```python
from build123d import *

# Parameters (mm, degrees)
SZKIC1_R                    = 4.5
DODANIE_WYCI_GNI_CIE1_DEPTH = 10
SZKIC3_R                    = 6.5
WYTNIJ_WYCI_GNI_CIE9_DEPTH  = 6.85
DODANIE_WYCI_GNI_CIE2_DEPTH = 18
DODANIE_WYCI_GNI_CIE3_DEPTH = 31.65
DODANIE_WYCI_GNI_CIE4_DEPTH = 20.5
WYTNIJ_WYCI_GNI_CIE3_REACH  = 73.312
SZKIC8_R                    = 1.7500000000000036
SZKIC8_R_2                  = 1.7499999999999982
SFAZOWANIE1_SIZE            = 2
DODANIE_WYCI_GNI_CIE5_DEPTH = 10
WYTNIJ_WYCI_GNI_CIE4_REACH  = 76.066
SZKIC12_R                   = 1.6000000000000019
WYTNIJ_WYCI_GNI_CIE6_START  = -5
SZKIC14_R                   = 7.499999999999999
WYTNIJ_WYCI_GNI_CIE6_DEPTH  = 5
SZKIC13_R                   = 4.000000000000001
WYTNIJ_WYCI_GNI_CIE5_DEPTH  = 1
ZAOKR_GLENIE1_R             = 2
ZAOKR_GLENIE2_R             = 1
WYTNIJ_WYCI_GNI_CIE7_DEPTH  = 13
WYTNIJ_WYCI_GNI_CIE8_REACH  = 71.325
SZKIC16_R                   = 1.599999999999998


with BuildPart() as part:
    # Szkic1 → Dodanie-wyciągnięcie1 (new body)
    with BuildSketch(Plane(origin=(0, 0, 0), x_dir=(1, 0, 0), z_dir=(0, 1, 0))):
        Polygon((-39.699999999999996, 14.25), (11.950000000000069, 14.25), (18.7, 7.5), (18.7, -7.5), (11.95000000000007, -14.25), (-39.699999999999996, -14.25), align=None)
        with Locations(Location((0, 0, 0), (0, 0, 270))):
            Circle(SZKIC1_R, mode=Mode.SUBTRACT)
    extrude(amount=DODANIE_WYCI_GNI_CIE1_DEPTH)

    # Szkic3 → Wytnij-wyciągnięcie9 (cut)
    with BuildSketch(Plane.XZ):
        with Locations(Location((0, 0, 0), (0, 0, 270))):
            Circle(SZKIC3_R)
    extrude(amount=-WYTNIJ_WYCI_GNI_CIE9_DEPTH, mode=Mode.SUBTRACT)

    # Szkic4 → Dodanie-wyciągnięcie2 (add)
    with BuildSketch(Plane(origin=(0, 10, 0), x_dir=(1, 0, 0), z_dir=(0, 1, 0))):
        Polygon((-39.699999999999996, 14.25), (-15, 14.25), (-14.999999999999996, -14.25), (-39.699999999999996, -14.25), align=None)
    extrude(amount=DODANIE_WYCI_GNI_CIE2_DEPTH)

    # Szkic6 → Dodanie-wyciągnięcie3 (add)
    with BuildSketch(Plane(origin=(0, 27.999999999999996, 0), x_dir=(1, 0, 0), z_dir=(0, 1, 0))):
        Polygon((-39.699999999999996, 14.25), (18.699999999999996, 14.25), (18.7, 10.25), (-39.699999999999996, 10.25), align=None)
    extrude(amount=DODANIE_WYCI_GNI_CIE3_DEPTH)

    # Szkic7 → Dodanie-wyciągnięcie4 (add)
    with BuildSketch(Plane.XY.offset(-10.25)):
        Polygon((18.7, 57.49999999999999), (10.499999999999995, 57.49999999999999), (10.499999999999996, 47.49999999999999), (18.7, 47.49999999999999), align=None)
        Polygon((-39.699999999999996, 57.499999999999986), (-31.000000000000007, 57.499999999999986), (-31.000000000000004, 47.499999999999986), (-39.699999999999996, 47.499999999999986), align=None)
    extrude(amount=DODANIE_WYCI_GNI_CIE4_DEPTH)

    # Szkic8 → Wytnij-wyciągnięcie3 (cut, up to next)
    with BuildSketch(Plane(origin=(0, 57.499999999999986, 0), x_dir=(1, 0, 0), z_dir=(0, 1, 0)), mode=Mode.PRIVATE) as wytnij_wyci_gni_cie3_sk1:
        with Locations(Location((-34.5, 5.450000000000001, 0), (0, 0, 270))):
            Circle(SZKIC8_R)
    wytnij_wyci_gni_cie3_tool1 = extrude(wytnij_wyci_gni_cie3_sk1.sketch, amount=-WYTNIJ_WYCI_GNI_CIE3_REACH, mode=Mode.PRIVATE) & part.part
    # Szkic8 → Wytnij-wyciągnięcie3 (cut, up to next)
    with BuildSketch(Plane(origin=(0, 57.499999999999986, 0), x_dir=(1, 0, 0), z_dir=(0, 1, 0)), mode=Mode.PRIVATE) as wytnij_wyci_gni_cie3_sk2:
        with Locations(Location((14.5, 5.450000000000002, 0), (0, 0, 270))):
            Circle(SZKIC8_R_2)
    wytnij_wyci_gni_cie3_tool2 = extrude(wytnij_wyci_gni_cie3_sk2.sketch, amount=-WYTNIJ_WYCI_GNI_CIE3_REACH, mode=Mode.PRIVATE) & part.part
    # Szkic8 → Wytnij-wyciągnięcie3 (cut, up to next)
    with BuildSketch(Plane(origin=(0, 57.499999999999986, 0), x_dir=(1, 0, 0), z_dir=(0, 1, 0)), mode=Mode.PRIVATE) as wytnij_wyci_gni_cie3_sk3:
        with Locations(Location((14.5, -5.450000000000002, 0), (0, 0, 270))):
            Circle(SZKIC8_R_2)
    wytnij_wyci_gni_cie3_tool3 = extrude(wytnij_wyci_gni_cie3_sk3.sketch, amount=-WYTNIJ_WYCI_GNI_CIE3_REACH, mode=Mode.PRIVATE) & part.part
    # Szkic8 → Wytnij-wyciągnięcie3 (cut, up to next)
    with BuildSketch(Plane(origin=(0, 57.499999999999986, 0), x_dir=(1, 0, 0), z_dir=(0, 1, 0)), mode=Mode.PRIVATE) as wytnij_wyci_gni_cie3_sk4:
        with Locations(Location((-34.5, -5.450000000000001, 0), (0, 0, 270))):
            Circle(SZKIC8_R)
    wytnij_wyci_gni_cie3_tool4 = extrude(wytnij_wyci_gni_cie3_sk4.sketch, amount=-WYTNIJ_WYCI_GNI_CIE3_REACH, mode=Mode.PRIVATE) & part.part
    add(wytnij_wyci_gni_cie3_tool1.solids().sort_by_distance((-34.5, 57.5, -5.45))[0], mode=Mode.SUBTRACT)
    add(wytnij_wyci_gni_cie3_tool2.solids().sort_by_distance((14.5, 57.5, -5.45))[0], mode=Mode.SUBTRACT)
    add(wytnij_wyci_gni_cie3_tool3.solids().sort_by_distance((14.5, 57.5, 5.45))[0], mode=Mode.SUBTRACT)
    add(wytnij_wyci_gni_cie3_tool4.solids().sort_by_distance((-34.5, 57.5, 5.45))[0], mode=Mode.SUBTRACT)

    # Sfazowanie1
    sfazowanie1_edges = [part.edges().sort_by_distance(p)[0] for p in [
        (-39.699999999999996, 29.824999999999996, -14.25),
        (-39.699999999999996, 14, 14.25),
        (18.699999999999996, 43.824999999999996, -14.25),
    ]]
    chamfer(sfazowanie1_edges, length=SFAZOWANIE1_SIZE)

    # Szkic9 → Dodanie-wyciągnięcie5 (add)
    with BuildSketch(Plane.XZ):
        with BuildLine():
            Line((18.7, -7.5), (11.950000000000069, -14.25))
            Line((11.950000000000069, -14.25), (4.326136457566238, -14.249999999999998))
            ThreePointArc((4.326136457566238, -14.249999999999998), (12.732322327669147, -18.59179734698027), (18.7, -11.25))
            Line((18.7, -11.25), (18.7, -7.5))
        make_face()
        with BuildLine():
            Line((18.7, 7.5), (18.7, 11.25))
            ThreePointArc((18.7, 11.25), (12.732322327669147, 18.59179734698027), (4.326136457566238, 14.249999999999998))
            Line((4.326136457566238, 14.249999999999998), (11.950000000000069, 14.25))
            Line((11.950000000000069, 14.25), (18.7, 7.5))
        make_face()
    extrude(amount=-DODANIE_WYCI_GNI_CIE5_DEPTH)

    # Szkic12 → Wytnij-wyciągnięcie4 (cut, up to next)
    with BuildSketch(Plane.XZ, mode=Mode.PRIVATE) as wytnij_wyci_gni_cie4_sk1:
        with Locations(Location((11.199999999999998, -11.25, 0), (0, 0, 270))):
            Circle(SZKIC12_R)
    wytnij_wyci_gni_cie4_tool1 = extrude(wytnij_wyci_gni_cie4_sk1.sketch, amount=-WYTNIJ_WYCI_GNI_CIE4_REACH, mode=Mode.PRIVATE) & part.part
    # Szkic12 → Wytnij-wyciągnięcie4 (cut, up to next)
    with BuildSketch(Plane.XZ, mode=Mode.PRIVATE) as wytnij_wyci_gni_cie4_sk2:
        with Locations(Location((11.199999999999998, 11.25, 0), (0, 0, 90))):
            Circle(SZKIC12_R)
    wytnij_wyci_gni_cie4_tool2 = extrude(wytnij_wyci_gni_cie4_sk2.sketch, amount=-WYTNIJ_WYCI_GNI_CIE4_REACH, mode=Mode.PRIVATE) & part.part
    add(wytnij_wyci_gni_cie4_tool1.solids().sort_by_distance((11.2, 0, -11.25))[0], mode=Mode.SUBTRACT)
    add(wytnij_wyci_gni_cie4_tool2.solids().sort_by_distance((11.2, 0, 11.25))[0], mode=Mode.SUBTRACT)

    # Szkic14 → Wytnij-wyciągnięcie6 (cut)
    with BuildSketch(Plane(origin=(0, 10, 0), x_dir=(1, 0, 0), z_dir=(0, 1, 0)).offset(WYTNIJ_WYCI_GNI_CIE6_START)):
        with Locations((11.199999999999998, -11.25)):
            Circle(SZKIC14_R)
        with Locations((11.199999999999998, 11.25)):
            Circle(SZKIC14_R)
    extrude(amount=WYTNIJ_WYCI_GNI_CIE6_DEPTH, mode=Mode.SUBTRACT)

    # Szkic13 → Wytnij-wyciągnięcie5 (cut)
    with BuildSketch(Plane(origin=(0, 5, 0), x_dir=(1, 0, 0), z_dir=(0, 1, 0))):
        with Locations(Location((11.199999999999998, 11.25, 0), (0, 0, 270))):
            Circle(SZKIC13_R)
        with Locations(Location((11.199999999999998, -11.25, 0), (0, 0, 90))):
            Circle(SZKIC13_R)
    extrude(amount=-WYTNIJ_WYCI_GNI_CIE5_DEPTH, mode=Mode.SUBTRACT)

    # Zaokrąglenie1
    zaokr_glenie1_edges = [part.edges().sort_by_distance(p)[0] for p in [
        (18.700000000000003, 7.5, 11.25),
        (18.7, 7.5, -11.25),
    ]]
    fillet(zaokr_glenie1_edges, radius=ZAOKR_GLENIE1_R - 0.0001)  # a hair under: the kernel refuses the full size

    # Zaokrąglenie2
    zaokr_glenie2_edges = [part.edges().sort_by_distance(p)[0] for p in [
        (4.326136457566238, 7.5, 14.25),
        (4.326136457566238, 7.5, -14.249999999999998),
    ]]
    fillet(zaokr_glenie2_edges, radius=ZAOKR_GLENIE2_R)

    # Szkic15 → Wytnij-wyciągnięcie7 (cut)
    with BuildSketch(Plane.ZY.offset(39.699999999999996)):
        Polygon((-10.25, 27.999999999999996), (10.25, 27.999999999999996), (10.250000000000002, 6), (-10.25, 6), align=None)
    extrude(amount=-WYTNIJ_WYCI_GNI_CIE7_DEPTH, mode=Mode.SUBTRACT)

    # Szkic16 → Wytnij-wyciągnięcie8 (cut, up to next)
    with BuildSketch(Plane(origin=(0, 6, 0), x_dir=(1, 0, 0), z_dir=(0, 1, 0)), mode=Mode.PRIVATE) as wytnij_wyci_gni_cie8_sk1:
        with Locations(Location((-33.2, 0, 0), (0, 0, 270))):
            Circle(SZKIC16_R)
    wytnij_wyci_gni_cie8_tool1 = extrude(wytnij_wyci_gni_cie8_sk1.sketch, amount=-WYTNIJ_WYCI_GNI_CIE8_REACH, mode=Mode.PRIVATE) & part.part
    add(wytnij_wyci_gni_cie8_tool1.solids().sort_by_distance((-33.2, 6, 0))[0], mode=Mode.SUBTRACT)


solid = part.part
```
For this review, take the finished solid that the model builds, in its own axes (mm). A direction names the side the tool comes from. Coordinates: 2 decimals unless noted, no trailing zeros. Write each loop counter-clockwise with the first axis right and the second up, starting at its lowest first coordinate (ties: lowest second). Pieces come first, ordered by that corner, then holes. Notation, with made-up numbers: (84.5, 83) - (92.5, 83) arc R16 cw to (92.5, 99) - close; hole circle Ø7 at (25, 43.25). An arc over 180 degrees is marked (long way). Put each result on its own line as item: value.
1. Add section B-B, the plane x = 0. Give the boundary of the cut face in (y, z), then the cut area to 3 significant figures.
Values found:
outline: (0, -14.25) - (10, -14.25) - (10, -4.5) - (6.85, -4.5) - (6.85, -6.5) - (0, -6.5) - close; (0, 6.5) - (6.85, 6.5) - (6.85, 4.5) - (10, 4.5) - (10, 14.25) - (0, 14.25) - close; (28, -14.25) - (59.65, -14.25) - (59.65, -10.25) - (28, -10.25) - close
area: 294 mm²
2. Wall thickness on probe 1 along X at (y, z) = (53.75, -5.45); probe 2 along Z at (x, y) = (14, 52); probe 3 along Z at (x, y) = (11, 1): over which ranges is each line inside the solid? List them lowest first.
Values found:
probe 1: -39.7 to -36.25, -32.75 to -31, 10.5 to 12.75, 16.25 to 18.7
probe 2: -14.25 to -7.13, -3.77 to 3.77, 7.13 to 10.25
probe 3: -18.75 to -12.84, -9.66 to 9.66, 12.84 to 18.75
3. Mouldability with a two-part tool opening along Z and no side actions: class faces 5 (the cylindrical face through (7.295, 4.507, -12.117)), 6 (the flat face through (18.7, 4, 0)), 7 (the flat face through (-38.71, 29.41, -13.24)) as released by +Z, released by -Z, zero draft, split by the parting line, or undercut.
Values found:
face 5: undercut
face 6: zero draft
face 7: released by -Z
4. Add section A-A, the plane z = 0. Give the boundary of the cut face in (x, y), then the cut area to 3 significant figures.
Values found:
outline: (-39.7, 0) - (-34.8, 0) - (-34.8, 6) - (-39.7, 6) - close; (-39.7, 47.5) - (-31, 47.5) - (-31, 57.5) - (-39.7, 57.5) - close; (-31.6, 0) - (-6.5, 0) - (-6.5, 6.85) - (-4.5, 6.85) - (-4.5, 10) - (-15, 10) - (-15, 28) - (-26.7, 28) - (-26.7, 6) - (-31.6, 6) - close; (4.5, 6.85) - (6.5, 6.85) - (6.5, 0) - (18.7, 0) - (18.7, 10) - (4.5, 10) - close; (10.5, 47.5) - (18.7, 47.5) - (18.7, 57.5) - (10.5, 57.5) - close
area: 775 mm²
5. For pin 1 (4 mm diameter, centred on y = 27, z = -2.5, fed in from +X); pin 2 (6 mm diameter, centred on x = -19.5, z = 2, fed in from +Y); pin 3 (4 mm diameter, centred on x = 6, z = 1, fed in from +Y), all flat-tipped, find the tip position at first contact; note any pin that passes through.
Values found:
pin 1: x = -15
pin 2: y = 28
pin 3: y = 10
6. Machinability: for faces 1 (the flat face through (-21, 11, 14.25)), 2 (the cylindrical face through (15.976, 52.57, 6.391)), 3 (the flat face through (-35, 53, 10.25)), 4 (the cylindrical face through (-3.955, 3.377, 5.158)), which of the approach directions +Z, -Z, +X, -X, +Y, -Y give a long, thin tool a straight path to every point of the face, cutting with its end or side? Answer none if there is none.
Values found:
face 1: +Z, -X, +Y, -Y
face 2: +Y
face 3: +Z, +X, -X, +Y
face 4: -Y
7. Add section D-D, the plane y = 38. Give the boundary of the cut face in (x, z).
Values found:
outline: (-39.7, -12.25) - (-37.7, -14.25) - (16.7, -14.25) - (18.7, -12.25) - (18.7, -10.25) - (-39.7, -10.25) - close
8. Add section C-C, the plane x = -24. Give the boundary of the cut face in (y, z).
Values found:
outline: (0, -14.25) - (59.65, -14.25) - (59.65, -10.25) - (28, -10.25) - (28, 14.25) - (0, 14.25) - close
